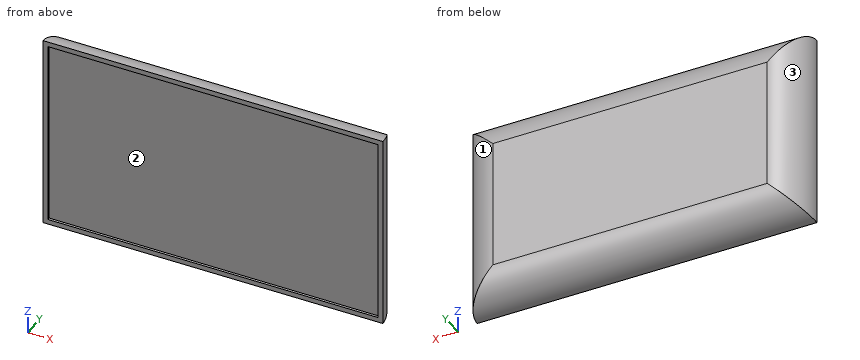
```python
from build123d import *

# Parameters (mm, degrees)
F0_W     = 263.9645430735
F0_H     = 152.4
F1_DEPTH = 25.4
F2_W     = 256.3445430735
F2_H     = 144.78
F3_DEPTH = 1.905
F4_R     = 25.39999


# Not quite as in the source:
# - a fillet or chamfer is up to 0.001 mm smaller than in the source, because OpenCascade refuses the exact size


with BuildPart() as f1:
    # F0 (on Front) → F1 (new body)
    with BuildSketch(Plane.XZ):
        with Locations((-0.0032023633, -16.0101552037)):
            Rectangle(F0_W, F0_H)
    extrude(amount=F1_DEPTH)

    # F2 (on face) → F3 (cut)
    with BuildSketch(Plane.XZ.offset(25.4)):
        with Locations((-0.0032023633, -16.0101552037)):
            Rectangle(F2_W, F2_H)
    extrude(amount=-F3_DEPTH, mode=Mode.SUBTRACT)

    # F4 (radius 25.4 in the source; OpenCascade refuses exactly that, so slightly less here)
    f4_edges = [f1.edges().sort_by_distance(p)[0] for p in [
        (-0.003202, 0, -92.210155),
        (131.979069, 0, -16.010155),
        (-0.003202, 0, 60.189845),
        (-131.985474, 0, -16.010155),
    ]]
    fillet(f4_edges, radius=F4_R)


solid = f1.part
```
Design review of the part built by this model. Coordinates are the model's own, in mm. Face numbers are marked on the shaded views. Coordinates: 2 decimals unless noted, no trailing zeros. Loops run counter-clockwise (first coordinate to the right, second up) from the corner with the lowest first, then second, coordinate; pieces in that order, holes last.
Q1. The part is to be moulded in two halves that separate along X. For the marked faces 1, 2 and 3, say which applies: +X half, -X half, draft (parallel to the pull), parting line (faces both ways), or undercut.
Reported:
face 1: +X half
face 2: undercut
face 3: -X half
Q2. For pin 1 (12 mm diameter, centred on x = -80, y = -5.5, fed in from +Z); pin 2 (1.5 mm diameter, centred on x = 5.5, y = -21, fed in from +Z); pin 3 (5 mm diameter, centred on y = -16.5, z = -50.5, fed in from +X), all flat-tipped, find the tip position at first contact; note any pin that passes through.
Reported:
pin 1: stops at z = 56.05
pin 2: stops at z = 59.93
pin 3: stops at x = 131.16
Q3. We need section D-D on y = -5. State the section outline as (x, z) points.
Reported:
outline: (-121.72, -81.94) - (121.71, -81.94) - (121.71, 49.92) - (-121.72, 49.92) - close
Q4. To check wall thickness, follow line 1 (Y direction, x = -73, z = -18.5) (3 decimals); line 2 (Z direction, x = 3.5, y = -8.75); line 3 (Z direction, x = 83, y = -11.5). State the ranges of each line that lie inside material, in increasing order.
Reported:
line 1: y = -23.495 to 0
line 2: z = -85.99 to 53.97
line 3: z = -88.07 to 56.05
Q5. We need section C-C on y = -17. State the section outline as (x, z) points, and give its area (3 significant figures).
Reported:
outline: (-130.56, -90.78) - (130.55, -90.78) - (130.55, 58.76) - (-130.56, 58.76) - close
area: 39,000 mm2
